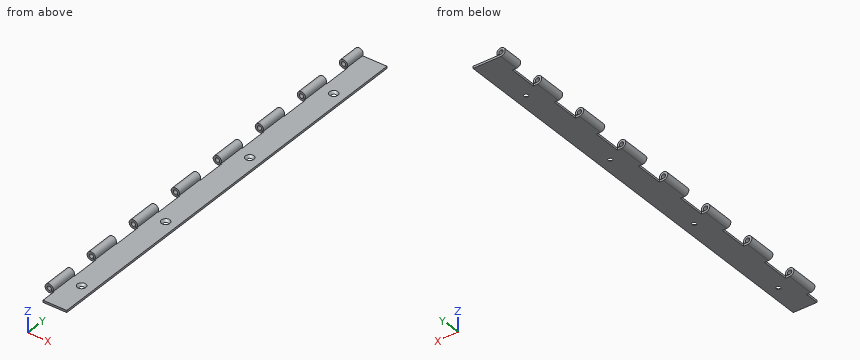
Autodesk Inventor part; units mm, degrees
ref_plane "YZ Plane" through (0, 0, 0) normal (1, 0, 0) x (0, 1, 0)
ref_plane "XZ Plane" through (0, 0, 0) normal (0, 1, 0) x (-1, 0, 0)
ref_plane "XY Plane" through (0, 0, 0) normal (0, 0, 1) x (1, 0, 0)
sketch "Sketch2" plane through (0, 0, 0) normal (0, 1, 0) x (-1, 0, 0)
  arc A0 (0, -1.5) -> (-1.3365, -0.681) centre (0, 0) ccw
  arc A1 (0, -3) -> (-2.673, -1.362) centre (0, 0) ccw
  line L0 (0, -3) -> (-20, -3)
  line L1 (-20, -3) -> (-20, -1.5)
  line L2 (-20, -1.5) -> (0, -1.5)
  line L3 (-1.3365, -0.681) -> (-2.673, -1.362)
  dimension "d0" = 1.5
  dimension "d1" = 1.5
  dimension "d2" = 20
  dimension "d3" = 3
  dimension "d4" = 27
extrude "Extrusion1" add sketch "Sketch2" along normal blind 304.8
sketch "Sketch3" plane through (20, 0, -3) normal (0, 0, -1) x (-1, 0, 0)
  line L0 (0, 0) -> (20, 0)
  line L1 (23, 50) -> (17, 50)
  line L2 (17, 50) -> (17, 30)
  line L3 (17, 30) -> (23, 30)
  line L4 (23, 30) -> (23, 50)
  line L5 (17, 0) -> (17, 304.8)
  dimension "d8" = 20
  dimension "d9" = 6
  dimension "d24" = 30
extrude "Extrusion2" cut sketch "Sketch3" against normal through all
pattern_linear "Rectangular Pattern1" count 25 spacing 40 along (0, 1, 0) of "Extrusion2"
sketch "Sketch5" plane through (20, 0, -3) normal (0, 0, -1) x (-1, 0, 0)
  line L0 (0, 0) -> (20, 0)
  line L1 (17, 0) -> (23, 0)
  line L2 (23, 0) -> (23, 10)
  line L3 (23, 10) -> (17, 10)
  line L4 (17, 10) -> (17, 0)
  point P0 (17, 30)
  dimension "d25" = 10
  dimension "d26" = 6
extrude "Extrusion3" cut sketch "Sketch5" against normal through all
sketch "Sketch4" plane through (20, 0, -1.5) normal (0, 0, 1) x (1, 0, 0)
  line L0 (0, 0) -> (0, 304.8)
  line L1 (0, 304.8) -> (-20, 304.8)
  point P0 (-8, -615.2)
  point P1 (-8, -535.2)
  point P2 (-8, -455.2)
  point P3 (-8, -375.2)
  point P4 (-8, -295.2)
  point P5 (-8, -215.2)
  point P6 (-8, -135.2)
  point P7 (-8, -55.2)
  point P8 (-8, 24.8)
  point P9 (-8, 104.8)
  point P10 (-8, 184.8)
  point P11 (-8, 264.8)
  point P12 (-17, 1000)
  point P13 (-20, 304.8)
  dimension "d15" = 8
  dimension "d29" = 40
  dimension "d30" = 80
  dimension "d31" = 80
  dimension "d32" = 80
  dimension "d33" = 80
  dimension "d34" = 80
  dimension "d35" = 80
  dimension "d36" = 80
  dimension "d37" = 80
  dimension "d38" = 80
  dimension "d39" = 80
  dimension "d40" = 80
hole "Hole1" at (12, -615.2, -1.5) at (12, -535.2, -1.5) at (12, -455.2, -1.5) at (12, -375.2, -1.5) at (12, -295.2, -1.5) at (12, -215.2, -1.5) at (12, -135.2, -1.5) at (12, -55.2, -1.5) at (12, 24.8, -1.5) at (12, 104.8, -1.5) at (12, 184.8, -1.5) at (12, 264.8, -1.5) direction (0, 0, -1) diameter 3 end through all countersink diameter 6 countersink angle 90
equation "\"d1\" = d0"
properties part number "SIDE 2" material "Steel, Mild"
Here's how the part is built. I have some questions about the finished solid (model axes, mm). Round coordinates to 2 decimals unless told otherwise and drop trailing zeros. Loops run counter-clockwise (first coordinate to the right, second up) from the corner with the lowest first, then second, coordinate; pieces in that order, holes last. Notation, with made-up numbers: (28, 42) -> (47, 42) arc R20 cw to (47, 73) -> close; hole circle Ø9 at (52.5, -22.75). An arc over 180 degrees is marked (long way). Write each question's results on one line, items separated by ' | '.
(1) For P1, Ø3, axis at x = 13.5, z = 0.5, coming from the +Y side; P2, Ø1.5, axis at x = 9.5, y = 166.5, coming from the +Z side; P3, Ø3, axis at x = -1, z = 0, coming from the -Y side; P4, Ø1.2, axis at y = 4, z = -2, coming from the -X side, each with a flat end and sliding along its axis, tell me the tip position at first contact or that it passes through.
Worked answers:
P1: through | P2: z = -1.5 | P3: y = 10 | P4: x = 3
(2) If we section it at B-B, the plane y = 220: List the corners of the cut face in (x, z) for me, then the cut area to 3 significant figures.
Worked answers:
outline: (0, -3) -> (20, -3) -> (20, -1.5) -> (0, -1.5) arc R1.5 cw (long way) to (1.34, -0.68) -> (2.67, -1.36) arc R3 ccw (long way) to start | area: 47.5 mm2
(3) If we section it at C-C, the plane y = 125.5: List the corners of the cut face in (x, z) for me.
Worked answers:
outline: (3, -3) -> (20, -3) -> (20, -1.5) -> (3, -1.5) -> close
(4) If we section it at A-A, the plane x = 12: List the corners of the cut face in (y, z) for me, then the cut area to 3 significant figures.
Worked answers:
outline: (0, -3) -> (23.3, -3) -> (21.8, -1.5) -> (0, -1.5) -> close; (26.3, -3) -> (103.3, -3) -> (101.8, -1.5) -> (27.8, -1.5) -> close; (106.3, -3) -> (183.3, -3) -> (181.8, -1.5) -> (107.8, -1.5) -> close; (186.3, -3) -> (263.3, -3) -> (261.8, -1.5) -> (187.8, -1.5) -> close; (266.3, -3) -> (304.8, -3) -> (304.8, -1.5) -> (267.8, -1.5) -> close | area: 430 mm2
(5) If I drill on L1, parallel to X at y = 26, z = -0.4; L2, parallel to X at y = 151, z = -2.55; L3, parallel to Z at x = 11.75, y = 134, over which ranges is the centre line in solid material (lowest first)?
Worked answers:
L1: -2.97 to -1.45, 1.45 to 2.97 | L2: 3 to 20 | L3: -3 to -1.5
